```python
from build123d import *

# Parameters (mm, degrees)
F0_W     = 129.935503
F0_H     = 129.381798
F0_R     = 53.156474
F1_DEPTH = 254
F2_R     = 50.8


with BuildPart() as f1:
    # F0 (on Front) → F1 (new body)
    with BuildSketch(Plane.XZ):
        with Locations((5.537025, -1.107406)):
            Rectangle(F0_W, F0_H)
        Circle(F0_R, mode=Mode.SUBTRACT)
    extrude(amount=F1_DEPTH)

    # F2
    f2_edges = [f1.edges().sort_by_distance(p)[0] for p in [
        (70.504777, -127, 63.583493),
    ]]
    fillet(f2_edges, radius=F2_R)


solid = f1.part
```
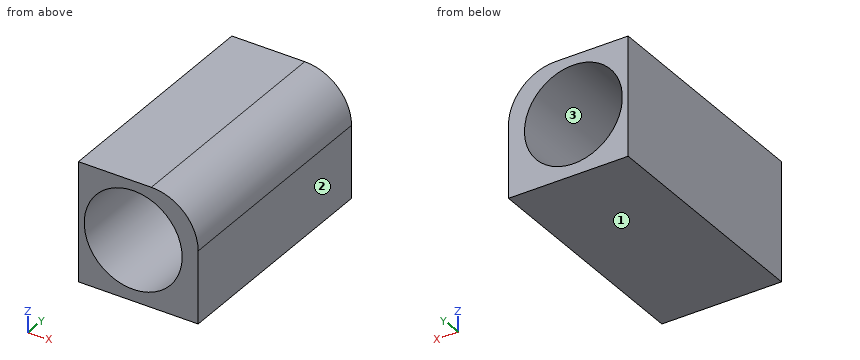
Model file for the job. Use its own axes, mm. Face numbers are marked on the shaded views. Give positions to 0.01 mm unless a question says otherwise; leave off trailing zeros. Write each loop counter-clockwise with the first axis right and the second up, starting at its lowest first coordinate (ties: lowest second). Pieces come first, ordered by that corner, then holes. Notation, with made-up numbers: (-22, -17) -> (-11, -17) arc R21 cw to (-11, -12) -> close; hole circle Ø1 at (-37, 4). An arc over 180 degrees is marked (long way). Use CSV: the item, a comma, the result in double quotes. Start each with the question number.
1) Two-plate mould, pull along X, no slides. Class the marked faces 1, 2 and 3: released by +X, released by -X, zero draft, split by the parting line, or undercut.
2) Drill centre lines: L1, parallel to Z at x = 0, y = -104; L2, parallel to Z at x = -2.5, y = -179; L3, parallel to X at y = -191.5, z = -24.5. Where is each one in solid material? Low to high.
3) Cut at D-D on x = 63.5. List the corners of the cut face in (y, z), plus the area to 3 significant figures.
4) Pin check, flat tips, straight feed: P1, Ø5, axis at x = 56.5, y = -145.5, coming from the +Z side; P2, Ø2, axis at x = 39.5, y = -44, coming from the +Z side. Stop position of each tip, or through.
5) Cut at B-B on y = -126. List the corners of the cut face in (x, z), plus the area to 3 significant figures.
6) Cut at C-C on x = 3.5. List the corners of the cut face in (y, z).
7) Cut at A-A on z = 0. List the corners of the cut face in (x, y).
Final values:
1,face 1,"zero draft"
1,face 2,"released by +X"
1,face 3,"undercut"
2,L1,"z = -65.8 to -53.16, 53.16 to 63.58"
2,L2,"z = -65.8 to -53.1, 53.1 to 63.58"
2,L3,"x = -59.43 to -47.17, 47.17 to 70.5"
3,outline,"(-254, -65.8) -> (0, -65.8) -> (0, 38.52) -> (-254, 38.52) -> close"
3,area,"26,500 mm2"
4,P1,"stops at z = 50.26"
4,P2,"stops at z = 59.98"
5,outline,"(-59.43, -65.8) -> (70.5, -65.8) -> (70.5, 12.78) arc R50.8 ccw to (19.7, 63.58) -> (-59.43, 63.58) -> close; hole circle Ø106.31 at (0, 0)"
5,area,"7,380 mm2"
6,outline,"(-254, -65.8) -> (0, -65.8) -> (0, -53.04) -> (-254, -53.04) -> close; (-254, 53.04) -> (0, 53.04) -> (0, 63.58) -> (-254, 63.58) -> close"
7,outline,"(-59.43, -254) -> (-53.16, -254) -> (-53.16, 0) -> (-59.43, 0) -> close; (53.16, -254) -> (70.5, -254) -> (70.5, 0) -> (53.16, 0) -> close"
